Read the model definition and answer for the solid it produces. Units are mm, in the model's axes. Face numbers are marked on the shaded views. A direction names the side the tool comes from. Round coordinates to 2 decimals unless told otherwise and drop trailing zeros. Loops run counter-clockwise (first coordinate to the right, second up) from the corner with the lowest first, then second, coordinate; pieces in that order, holes last. Notation, with made-up numbers: M 52,12.5 L 68,12.5 A15 cw 68,36.5 Z; hole C 61,12.5 d1. An arc over 180 degrees is marked long. Write each question's results on one line, items separated by ' | '.
```python
from build123d import *

# Parameters (mm, degrees)
F1_DEPTH = 61.9365051389
F2_R     = 29.6414431948
F3_DEPTH = 44.7673946619


with BuildPart() as f1:
    # F0 (on Front) → F1 (new body)
    with BuildSketch(Plane.XZ):
        with BuildLine():
            Line((86.4637133837, 104.3530513048), (35.6637133837, 104.3530513048))
            ThreePointArc((35.6637133837, 104.3530513048), (-0.2573111006, 89.4740757891), (-15.1362866163, 53.5530513048))
            Line((-15.1362866163, 53.5530513048), (-15.1362866163, -22.6469486952))
            Line((-15.1362866163, -22.6469486952), (86.4637133837, -22.6469486952))
            Line((86.4637133837, -22.6469486952), (86.4637133837, 104.3530513048))
        make_face()
    extrude(amount=F1_DEPTH)

    # F2 (on face) → F3 (join)
    with BuildSketch(Plane(origin=(0, 0, 0), x_dir=(-1, 0, 0), z_dir=(0, 1, 0))):
        with Locations((-36.5680158138, 40.3463989496)):
            Circle(F2_R)
    extrude(amount=F3_DEPTH)


solid = f1.part
```
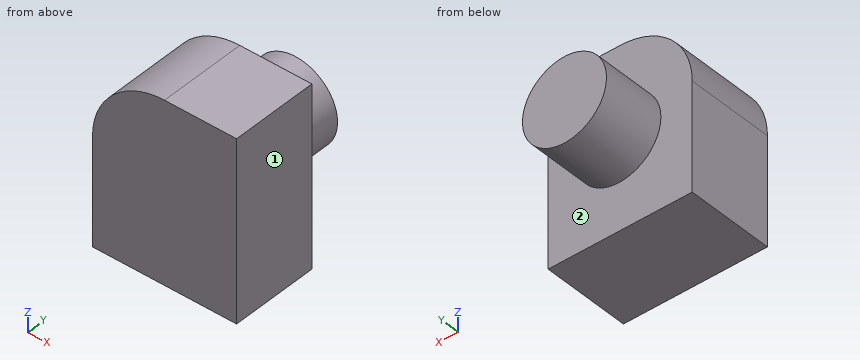
1. Which of the six approach directions +Z, -Z, +X, -X, +Y, -Y give full straight-line access (tool end or side, diameter ignored) to the marked faces 1 and 2?
Completed:
face 1: +Z, -Z, +X, +Y, -Y | face 2: +Y
2. Find section C-C, the plane z = 13.5. Give the vertices of the cut face in (x, y).
Completed:
outline: M -15.14,-61.94 L 86.46,-61.94 L 86.46,0 L 49.13,0 L 49.13,44.77 L 24,44.77 L 24,0 L -15.14,0 Z
3. Find section A-A, the plane y = -28. Give the vertices of the cut face in (x, z), then the cut area to 3 significant figures.
Completed:
outline: M -15.14,-22.65 L 86.46,-22.65 L 86.46,104.35 L 35.66,104.35 A50.8 ccw -15.14,53.55 Z | area: 12,300 mm2
4. Find section D-D, the plane x = -4.5. Give the vertices of the cut face in (y, z), then the cut area to 3 significant figures.
Completed:
outline: M -61.94,-22.65 L 0,-22.65 L 0,84.66 L -61.94,84.66 Z | area: 6,650 mm2
5. Find section B-B, the plane x = 41. Give the vertices of the cut face in (y, z).
Completed:
outline: M -61.94,-22.65 L 0,-22.65 L 0,11.04 L 44.77,11.04 L 44.77,69.65 L 0,69.65 L 0,104.35 L -61.94,104.35 Z
6. Given P1, Ø1.5, axis at x = 51, z = 80, coming from the +Y side; P2, Ø2, axis at x = 64.5, y = 19.5, coming from the +Z side; P3, Ø6, axis at x = 64, y = 14, coming from the +Z side, each flat-ended and moving along its own axis, determine where each tip first touches the part or whether it passes through.
Completed:
P1: stops at y = 0 | P2: stops at z = 52.73 | P3: stops at z = 57.13
7. Find the intervals of material crossed by L1, parallel to Y at x = 0.5, z = 87; L2, parallel to X at y = 11.5, z = 40; L3, parallel to Z at x = 34, y = -4.5, in increasing order.
Completed:
L1: y = -61.94 to 0 | L2: x = 6.93 to 66.21 | L3: z = -22.65 to 104.33
